Source: three-view drawing plus pictorial views. Frame: mm from the lowest corner of the part. A direction names the side the tool comes from. Give positions to 0.01 mm unless a question says otherwise; leave off trailing zeros. Loops run counter-clockwise (first coordinate to the right, second up) from the corner with the lowest first, then second, coordinate; pieces in that order, holes last. Notation, with made-up numbers: M -32,45.25 L 14,45.25 A32 cw 14,81.25 Z; hole C 21,28 d7. An arc over 180 degrees is marked long. One line per item, written item: value. Start each with the question number.
(1) Section C-C on x = 40. Output: boundary loops of the cut face in (y, z), plus the area to 3 significant figures.
(2) Section A-A on z = 4. Output: boundary loops of the cut face in (x, y).
(3) Ray query, line 1 along Z through (x, y) = (35, 26); line 2 along X through (y, z) = (26, 23.5); line 3 along Z through (x, y) = (40.5, 12). Return the intervals inside material, ascending. Write a range as from..to.
(4) Section B-B on y = 24. Output: boundary loops of the cut face in (x, z), plus the area to 3 significant figures.
(5) Pull-direction query (X, two-part tool) for the marked faces 4, 5 and 6; classes: released by +X, released by -X, zero draft, split by the parting line, or undercut.
(6) Access query for the marked faces 1, 2 and 3. Directions: +Z, -Z, +X, -X, +Y, -Y. A direction counts if a zero-diameter tool reaches every point of the face in a straight line with its end or side. Return the directions, or none.
(7) Pin query (flat end, axial travel): P1, Ø10, axis at x = 43.5, y = 6, coming from the -Z side; P2, Ø14, axis at y = 16.5, z = 27.5, coming from the +X side; P3, Ø4, axis at x = 24.5, y = 4, coming from the -Z side; P4, Ø10, axis at x = 47.5, y = 13, coming from the +Z side. Return the tip coordinate at first contact, or that it passes through.
(8) Section D-D on z = 20. Output: boundary loops of the cut face in (x, y), plus the area to 3 significant figures.
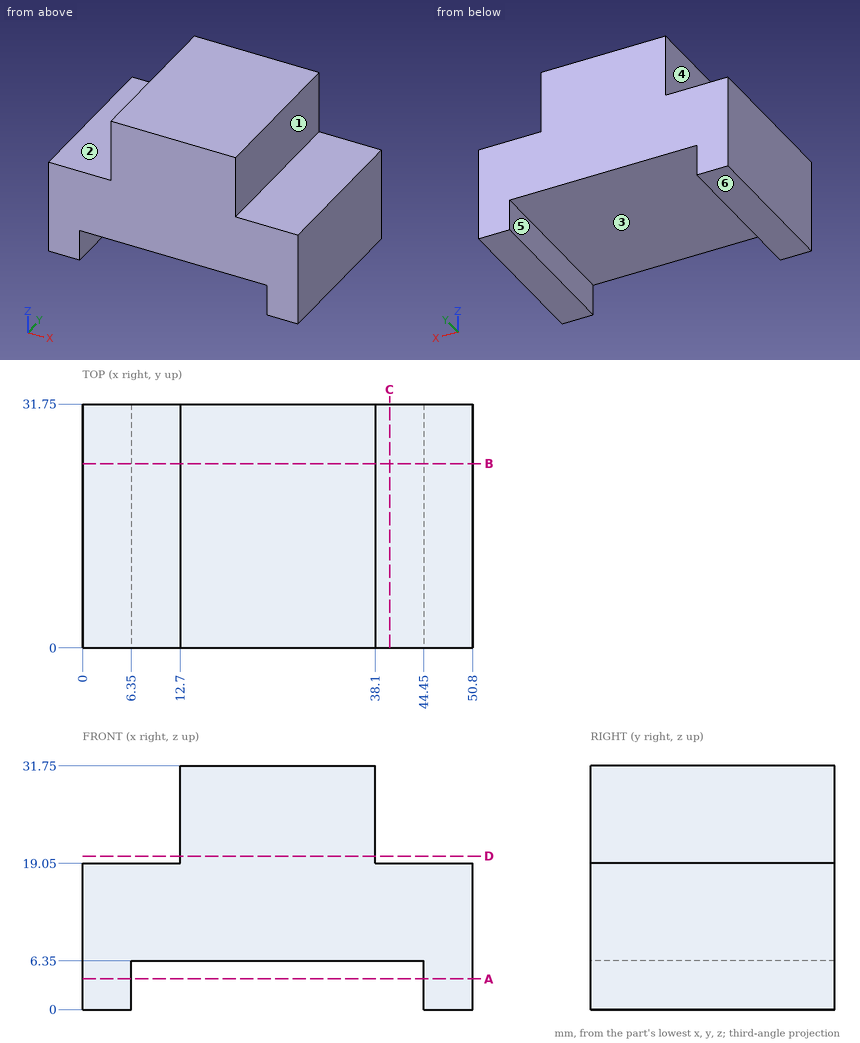
Output values:
1. outline: M 0,6.35 L 31.75,6.35 L 31.75,19.05 L 0,19.05 Z
1. area: 403 mm²
2. outline: M 0,0 L 6.35,0 L 6.35,31.75 L 0,31.75 Z; M 44.45,0 L 50.8,0 L 50.8,31.75 L 44.45,31.75 Z
3. line 1: z = 6.35..31.75
3. line 2: x = 12.7..38.1
3. line 3: z = 6.35..19.05
4. outline: M 0,0 L 6.35,0 L 6.35,6.35 L 44.45,6.35 L 44.45,0 L 50.8,0 L 50.8,19.05 L 38.1,19.05 L 38.1,31.75 L 12.7,31.75 L 12.7,19.05 L 0,19.05 Z
4. area: 1,050 mm²
5. face 4: released by -X
5. face 5: undercut
5. face 6: zero draft
6. face 1: +Z, +X, +Y, -Y
6. face 2: +Z, -X, +Y, -Y
6. face 3: -Z, +Y, -Y
7. P1: stops at z = 0
7. P2: stops at x = 38.1
7. P3: stops at z = 6.35
7. P4: stops at z = 19.05
8. outline: M 12.7,0 L 38.1,0 L 38.1,31.75 L 12.7,31.75 Z
8. area: 806 mm²
